Part model, mm, in its own coordinate system. A direction names the side the tool comes from. Round coordinates to 2 decimals unless told otherwise and drop trailing zeros. Loops run counter-clockwise (first coordinate to the right, second up) from the corner with the lowest first, then second, coordinate; pieces in that order, holes last.
1) Drop flat-ended pins along their axis: P1, Ø12, axis at x = 43.5, z = 607.5, coming from the -Y side; P2, Ø6, axis at y = -21.5, z = 402.5, coming from the +X side; P3, Ø5, axis at y = -26.5, z = 255, coming from the +X side. Give the stop position or say it passes through.
2) Mould opens along X. For faces 3 (the flat face through (29, 37.5, 345)), 4 (the flat face through (0, -34, 345)), 5 (the cylindrical face through (35.1, 34.3, 263.1)) say: +X half, -X half, draft (parallel to the pull), parting line (faces both ways), or undercut.
3) Band-saw the part on B-B, the plane y = -0.5. Write the cut outline in (x, z).
4) Probe line 1 (Y direction, x = 71.5, z = 598.5); line 2 (Z direction, x = 44, y = 32); line 3 (X direction, y = 30.5, z = 616.5). List the from-to ranges inside material, lowest first.
5) 3-axis set-ups, long thin cutter, end or side, ignore diameter. For faces 1 (the cylindrical face through (41.39, 34.28, 355.53)), 2 (the flat face through (6.35, 0, 500)): which of +Z, -Z, +X, -X, +Y, -Y reach the whole face in a straight line?
6) Band-saw the part on C-C, the plane z = 46. Write the cut outline in (x, y), then the cut area to 3 significant figures.
7) Band-saw the part on A-A, the plane x = 65. Write the cut outline in (y, z).
from build123d import *

# Parameters (mm, degrees)
BOSS_EXTRUDE1_DEPTH = 700
SKETCH3_W           = 125
SKETCH3_H           = 60
CUT_EXTRUDE1_DEPTH  = 706.00443261
CHAMFER1_SIZE       = 30
SKETCH4_R           = 10
CUT_EXTRUDE2_DEPTH  = 708.990112925
SKETCH5_R           = 7.5
CUT_EXTRUDE3_DEPTH  = 708.990112925
CHAMFER2_SIZE       = 3
FILLET1_R           = 3


with BuildPart() as part:
    # Sketch1 → Boss-Extrude1 (new body)
    with BuildSketch(Plane.XY):
        Polygon((0, -37.5), (0, 37.5), (75, 37.5), (75, 31.15), (6.35, 31.15), (6.35, -31.15), (75, -31.15), (75, -37.5), align=None)
    extrude(amount=BOSS_EXTRUDE1_DEPTH)

    # Sketch3 → Cut-Extrude1 (cut, through all)
    with BuildSketch(Plane.ZY):
        with Locations((92.5, 0)):
            Rectangle(SKETCH3_W, SKETCH3_H)
        with Locations((607.5, 0)):
            Rectangle(SKETCH3_W, SKETCH3_H)
        Polygon((400, 10.383333333), (373, 10.383333333), (373, 31.15), (327, 31.15), (307, 31.15), (307, 10.383333333), (300, 10.383333333), (270, 10.383333333), (270, -10.383333333), (300, -10.383333333), (327, -10.383333333), (327, -31.15), (373, -31.15), (393, -31.15), (393, -10.383333333), (400, -10.383333333), align=None)
    extrude(amount=-CUT_EXTRUDE1_DEPTH, mode=Mode.SUBTRACT)

    # Chamfer1
    chamfer1_edges = [part.edges().sort_by_distance(p)[0] for p in [
        (75, -34.325, 0),
        (75, 34.325, 700),
        (75, -34.325, 700),
        (75, 34.325, 0),
    ]]
    chamfer(chamfer1_edges, length=CHAMFER1_SIZE)

    # Sketch4 → Cut-Extrude2 (cut, through all)
    with BuildSketch(Plane(origin=(0, 37.5, 0), x_dir=(1, 0, 0), z_dir=(0, 1, 0))):
        with Locations(Location((43.5, -607.5, 0), (0, 0, 270))):
            Circle(SKETCH4_R)
        with Locations(Location((43.5, -92.5, 0), (0, 0, 270))):
            Circle(SKETCH4_R)
    extrude(amount=-CUT_EXTRUDE2_DEPTH, mode=Mode.SUBTRACT)

    # Sketch5 → Cut-Extrude3 (cut, through all)
    with BuildSketch(Plane.XZ.offset(37.5)):
        with Locations(Location((38, 270.017579968, 0), (0, 0, 270))):
            Circle(SKETCH5_R)
        with Locations(Location((36.322953254, 350, 0), (0, 0, 270))):
            Circle(SKETCH5_R)
    extrude(amount=-CUT_EXTRUDE3_DEPTH, mode=Mode.SUBTRACT)

    # Chamfer2
    chamfer2_edges = [part.edges().sort_by_distance(p)[0] for p in [
        (6.35, 0, 155),
        (6.35, 0, 545),
        (6.35, -20.766666667, 327),
        (6.35, 0, 270),
        (6.35, 20.766666667, 373),
        (0, -20.766666667, 393),
        (0, 20.766666667, 307),
    ]]
    chamfer(chamfer2_edges, length=CHAMFER2_SIZE)

    # Fillet1
    fillet1_edges = [part.edges().sort_by_distance(p)[0] for p in [
        (1.675, 10.383333333, 270),
        (1.675, -10.383333333, 270),
        (1.675, 31.15, 373),
        (1.675, -31.15, 327),
        (4.675, -31.15, 393),
        (4.675, 31.15, 307),
        (3.175, 10.383333333, 400),
        (3.175, -10.383333333, 400),
    ]]
    fillet(fillet1_edges, radius=FILLET1_R)


solid = part.part
Reported:
1. P1: passes through
1. P2: stops at x = 6.35
1. P3: stops at x = 6.35
2. face 3: draft
2. face 4: -X half
2. face 5: undercut
3. outline: (0, 0) - (6.35, 0) - (6.35, 30) - (0, 30) - close; (0, 155) - (3.35, 155) - (6.35, 158) - (6.35, 267) - (3.35, 270) - (0, 270) - close; (0, 400) - (6.35, 400) - (6.35, 542) - (3.35, 545) - (0, 545) - close; (0, 670) - (6.35, 670) - (6.35, 700) - (0, 700) - close
4. line 1: y = -37.5 to -31.15, 31.15 to 37.5
4. line 2: z = 0 to 82.51, 102.49 to 265.52, 274.52 to 597.51, 617.49 to 700
4. line 3: x = 0 to 6.35
5. face 1: +Y, -Y
5. face 2: +Z, -Z, +X
6. outline: (0, -37.5) - (75, -37.5) - (75, -31.15) - (6.35, -31.15) - (6.35, -30) - (0, -30) - close; (0, 30) - (6.35, 30) - (6.35, 31.15) - (75, 31.15) - (75, 37.5) - (0, 37.5) - close
6. area: 967 mm2
7. outline: (-37.5, 20) - (-31.15, 20) - (-31.15, 680) - (-37.5, 680) - close; (31.15, 20) - (37.5, 20) - (37.5, 680) - (31.15, 680) - close
